Work out the finished part from the listing and answer in its coordinate system (mm). Round coordinates to 2 decimals unless told otherwise and drop trailing zeros. Write each loop counter-clockwise with the first axis right and the second up, starting at its lowest first coordinate (ties: lowest second). Pieces come first, ordered by that corner, then holes. Notation, with made-up numbers: M 53.25,16.5 L 85.25,16.5 A17 ccw 85.25,48.5 Z; hole C 35,82 d11. An arc over 180 degrees is marked long. Answer in a Markdown table with one row per item.
```python
from build123d import *

# Parameters (mm, degrees)
ESQUISSE1_R        = 2
BOSS_EXTRU_1_DEPTH = 4


with BuildPart() as part:
    # Esquisse1 → Boss.-Extru.1 (new body)
    with BuildSketch(Plane.XY):
        with BuildLine():
            Line((0, 5), (40, 5))
            ThreePointArc((40, 5), (45, 0), (40, -5))
            Line((40, -5), (0, -5))
            ThreePointArc((0, -5), (-5, 0), (0, 5))
        make_face()
        with Locations((40, 0)):
            Circle(ESQUISSE1_R, mode=Mode.SUBTRACT)
        Circle(ESQUISSE1_R, mode=Mode.SUBTRACT)
    extrude(amount=BOSS_EXTRU_1_DEPTH)


solid = part.part
```
1. The part is cut by section D-D (y = -3.5). Determine the outline of the cut face in (x, z), plus the area to 3 significant figures.
Calculated:
| item | result |
|---|---|
| outline | M -3.57,0 L 43.57,0 L 43.57,4 L -3.57,4 Z |
| area | 189 mm² |
2. The part is cut by section A-A (y = 0). Determine the outline of the cut face in (x, z).
Calculated:
| item | result |
|---|---|
| outline | M -5,0 L -2,0 L -2,4 L -5,4 Z; M 2,0 L 38,0 L 38,4 L 2,4 Z; M 42,0 L 45,0 L 45,4 L 42,4 Z |
3. Consider line 1 along Y through (x, z) = (0, 1.95); line 2 along X through (y, z) = (-1.75, 0.9); line 3 along X through (y, z) = (-3.5, 1.8). Determine where each line is inside the solid, lowest interval first. Write a range as from..to.
Calculated:
| item | result |
|---|---|
| line 1 | y = -5..-2, 2..5 |
| line 2 | x = -4.68..-0.97, 0.97..39.03, 40.97..44.68 |
| line 3 | x = -3.57..43.57 |
4. The part is cut by section B-B (x = -1). Determine the outline of the cut face in (y, z).
Calculated:
| item | result |
|---|---|
| outline | M -4.9,0 L -1.73,0 L -1.73,4 L -4.9,4 Z; M 1.73,0 L 4.9,0 L 4.9,4 L 1.73,4 Z |
5. The part is cut by section C-C (z = 1.05). Determine the outline of the cut face in (x, y).
Calculated:
| item | result |
|---|---|
| outline | M 0,-5 L 40,-5 A5 ccw 40,5 L 0,5 A5 ccw Z; hole C 0,0 d4; hole C 40,0 d4 |
6. Determine the mould class of faces 1 (the cylindrical face through (38, 0, 2)), 2 (the flat face through (20, 0, 4)), 3 (the cylindrical face through (45, 0, 2)), 4 (the flat face through (20, -5, 2)) for opening direction Y: released by +Y, released by -Y, zero draft, split by the parting line, or undercut.
Calculated:
| item | result |
|---|---|
| face 1 | undercut |
| face 2 | zero draft |
| face 3 | split by the parting line |
| face 4 | released by -Y |
7. Given pin 1 (1 mm diameter, centred on y = 2.5, z = 1, fed in from -X); pin 2 (4.5 mm diameter, centred on x = 40, y = 0, fed in from +Z), each flat-ended and moving along its own axis, determine where each tip first touches the part or whether it passes through.
Calculated:
| item | result |
|---|---|
| pin 1 | stops at x = -4.58 |
| pin 2 | stops at z = 4 |
